from build123d import *

# Parameters (mm, degrees)
SKETCH3_R               = 6.35
CUT_EXTRUDE1_DEPTH      = 32.75
CUT_EXTRUDE1_DEPTH_BACK = 45.45


with BuildPart() as part:
    # Sketch1 → Revolve1 (revolve)
    with BuildSketch(Plane(origin=(0, 0, 0), x_dir=(1, 0, 0), z_dir=(0, 1, 0))):
        with BuildLine():
            Line((-89.802561211, -38.1), (-57.15, -38.1))
            ThreePointArc((-57.15, -38.1), (-52.659871939, -36.240128061), (-50.8, -31.75))
            Line((-50.8, -31.75), (-50.8, 31.75))
            ThreePointArc((-50.8, 31.75), (-52.659871939, 36.240128061), (-57.15, 38.1))
            Line((-57.15, 38.1), (-89.802561211, 38.1))
            ThreePointArc((-89.802561211, 38.1), (-93.46873542, 36.934753289), (-95.789398625, 33.866666667))
            ThreePointArc((-95.789398625, 33.866666667), (-101.6, 0), (-95.789398625, -33.866666667))
            ThreePointArc((-95.789398625, -33.866666667), (-93.46873542, -36.934753289), (-89.802561211, -38.1))
        make_face()
    revolve(axis=Axis((0, 0, 0), (0, 0, 1)))

    # Sketch2 → Revolve2 (revolve)
    with BuildSketch(Plane(origin=(0, 0, 0), x_dir=(1, 0, 0), z_dir=(0, 1, 0))):
        Polygon((-44.45, 31.75), (-50.8, 31.75), (-50.8, -31.75), (-44.45, -31.75), (-44.45, -6.35), (0, -6.35), (0, 6.35), (-44.45, 6.35), align=None)
        with BuildLine():
            Line((-50.8, -31.75), (-50.8, 31.75))
            ThreePointArc((-50.8, 31.75), (-52.659871939, 36.240128061), (-57.15, 38.1))
            Line((-57.15, 38.1), (-89.802561211, 38.1))
            ThreePointArc((-89.802561211, 38.1), (-93.46873542, 36.934753289), (-95.789398625, 33.866666667))
            ThreePointArc((-95.789398625, 33.866666667), (-101.6, 0), (-95.789398625, -33.866666667))
            ThreePointArc((-95.789398625, -33.866666667), (-93.46873542, -36.934753289), (-89.802561211, -38.1))
            Line((-89.802561211, -38.1), (-57.15, -38.1))
            ThreePointArc((-57.15, -38.1), (-52.659871939, -36.240128061), (-50.8, -31.75))
        make_face()
    revolve(axis=Axis((0, 0, 0), (0, 0, 1)))

    # Sketch3 → Cut-Extrude1 (cut, two sides)
    with BuildSketch(Plane.XY.offset(6.35)) as cut_extrude1_sk:
        Circle(SKETCH3_R)
    extrude(amount=CUT_EXTRUDE1_DEPTH, mode=Mode.SUBTRACT)
    extrude(cut_extrude1_sk.sketch, amount=-CUT_EXTRUDE1_DEPTH_BACK, mode=Mode.SUBTRACT)


solid = part.part
Could you check a few things on this model? Use its own coordinates, in mm. A direction names the side the tool comes from. Give positions to 0.01 mm unless a question says otherwise; leave off trailing zeros. Write each loop counter-clockwise with the first axis right and the second up, starting at its lowest first coordinate (ties: lowest second). Pieces come first, ordered by that corner, then holes. Notation, with made-up numbers: (29.5, 28) -> (33.5, 28) arc R33 cw to (33.5, 62) -> close; hole circle Ø7 at (-4.75, 81). An arc over 180 degrees is marked (long way). Answer as a JSON object with one key per item and string values.
Q1. Suppose I cut it at C-C on z = -2.5. Write out the boundary of the cut face in (x, y).
Taken from the geometry:
{"outline": "circle Ø203.14 at (0, 0); hole circle Ø12.7 at (0, 0)"}
Q2. Will these pins go through, and if not, where does the flat tip stop? pin 1 Ø3 at (y, z) = (45.5, -1) entering from -X; pin 2 Ø8 at (x, z) = (33.5, -29.5) entering from -Y; pin 3 Ø8 at (y, z) = (37, 13.5) entering from +X.
Taken from the geometry:
{"pin 1": "stops at x = -91.57", "pin 2": "stops at y = -93.12", "pin 3": "stops at x = 95.24"}
Q3. Suppose I cut it at D-D on z = 24.5. Write out the boundary of the cut face in (x, y), then the cut area to 3 significant figures.
Taken from the geometry:
{"outline": "circle Ø197.2 at (0, 0); hole circle Ø88.9 at (0, 0)", "area": "24,300 mm²"}
Q4. Which directions (+Z, -Z, +X, -X, +Y, -Y) give clear straight access to the entire face, cutting with the end or side of a thin tool? Please do faces 1 (the flat face through (1, 59, 38.1)), 2 (the cylindrical face through (-42.397, -13.352, 18.872)), 3 (the flat face through (-1, 9, -6.35)).
Taken from the geometry:
{"face 1": "+Z, +X, -X, +Y, -Y", "face 2": "+Z", "face 3": "-Z"}
Q5. We'd pull the mould along X, two halves only. Please class faces 4 (the flat face through (-1, 59, -38.1)), 5 (the flat face through (0, 45, -31.75)): released by +X, released by -X, zero draft, split by the parting line, or undercut.
Taken from the geometry:
{"face 4": "zero draft", "face 5": "undercut"}
Q6. Please list where these lines run through material, in increasing order: L1, parallel to Y at x = 0, z = 1; L2, parallel to Z at x = -30.5, y = 34.5; L3, parallel to X at y = -24, z = -11.5.
Taken from the geometry:
{"L1": "y = -101.6 to -6.35, 6.35 to 101.6", "L2": "z = -31.75 to 31.75", "L3": "x = -98.05 to -37.41, 37.41 to 98.05"}
Q7. Suppose I cut it at A-A on x = 0. Write out the boundary of the cut face in (y, z), then the cut area to 3 significant figures.
Taken from the geometry:
{"outline": "(-95.79, -33.87) arc R6.35 ccw to (-89.8, -38.1) -> (-57.15, -38.1) arc R6.35 ccw to (-50.8, -31.75) -> (-44.45, -31.75) -> (-44.45, -6.35) -> (-6.35, -6.35) -> (-6.35, 6.35) -> (-44.45, 6.35) -> (-44.45, 31.75) -> (-50.8, 31.75) arc R6.35 ccw to (-57.15, 38.1) -> (-89.8, 38.1) arc R6.35 ccw to (-95.79, 33.87) arc R101.6 ccw to start; (6.35, -6.35) -> (44.45, -6.35) -> (44.45, -31.75) -> (50.8, -31.75) arc R6.35 ccw to (57.15, -38.1) -> (89.8, -38.1) arc R6.35 ccw to (95.79, -33.87) arc R101.6 ccw to (95.79, 33.87) arc R6.35 ccw to (89.8, 38.1) -> (57.15, 38.1) arc R6.35 ccw to (50.8, 31.75) -> (44.45, 31.75) -> (44.45, 6.35) -> (6.35, 6.35) -> close", "area": "9,100 mm²"}
